For this review, take the finished solid that the model builds, in its own axes (mm). A direction names the side the tool comes from. Give positions to 0.01 mm unless a question says otherwise; leave off trailing zeros. Loops run counter-clockwise (first coordinate to the right, second up) from the corner with the lowest first, then second, coordinate; pieces in that order, holes last. Notation, with made-up numbers: (17.5, -33.5) - (33.5, -33.5) arc R34 cw to (33.5, 5.5) - close; hole circle Ø9 at (33, 37). An arc over 180 degrees is marked (long way). Use CSV: the item, a comma, the result in double quotes. Start each with the question number.
1. For pin 1 (0.9 mm diameter, centred on x = 34, z = 1.5, fed in from -Y); pin 2 (1.5 mm diameter, centred on y = 3, z = 2, fed in from +X); pin 3 (0.9 mm diameter, centred on y = -29.5, z = 2, fed in from -X); pin 4 (8 mm diameter, centred on x = 16, y = 2.5, fed in from -Z), all flat-tipped, find the tip position at first contact; note any pin that passes through.
2. Take a section at C-C on y = 10.5. Give the boundary of the cut face in (x, z), plus the area to 3 significant figures.
3. For faces 4 (the flat face through (36, 7.5, 1)), 5 (the flat face through (-20, 30, 1)), 6 (the flat face through (-7.5, -52, 1)), 7 (the flat face through (25, -7, 1)), 8 (the flat face through (-35, -30, 1)), list the 3-axis set-ups (+Z, -Z, +X, -X, +Y, -Y) from which the entire face can be reached by the end or side of a thin tool; tool diameter is ignored.
4. Take a section at D-D on x = 20. Give the boundary of the cut face in (y, z).
5. Mouldability with a two-part tool opening along X and no side actions: class faces 1 (the flat face through (-37, -22.5, 1)), 2 (the flat face through (-5, -8, 1)), 3 (the flat face through (35, 0, 1)) as pulls with the +X half, pulls with the -X half, needs draft (parallel to the pull), parting line crosses it, or undercut.
6. Wall thickness on line 1 (X direction, y = 12, z = 1.1); line 2 (X direction, y = -30, z = 1.15); line 3 (X direction, y = 27, z = 0.65): over which ranges is each line inside the solid? List them lowest first.
7. Take a section at B-B on x = -20. Give the boundary of the cut face in (y, z).
8. Take a section at A-A on y = -5. Give the boundary of the cut face in (x, z), plus the area to 3 significant figures.
```python
from build123d import *

# Parameters (mm, degrees)
BOSS_EXTRUDE1_DEPTH = 3


with BuildPart() as part:
    # Sketch1 → Boss-Extrude1 (new body)
    with BuildSketch(Plane.XY):
        Polygon((35, 50), (-3, 30), (-38, 30), (-38, 7.5), (-35, 7.5), (-35, -7.5), (-38, -7.5), (-38, -22.5), (-35, -22.5), (-35, -37.5), (-38, -37.5), (-38, -50), (-27.5, -50), (-27.5, -53), (-7.5, -53), (-7.5, -50), (7.5, -50), (7.5, -53), (27.5, -53), (27.5, -50), (38, -50), (38, -37.5), (35, -37.5), (35, -22.5), (38, -22.5), (38, -7.5), (35, -7.5), (35, 7.5), (38, 7.5), (38, 22.5), (35, 22.5), (35, 37.5), (38, 37.5), (38, 50), align=None)
        with BuildLine():
            Line((-15, 20), (-15, -35))
            ThreePointArc((-15, -35), (-20, -40), (-25, -35))
            Line((-25, -35), (-25, 20))
            ThreePointArc((-25, 20), (-20, 25), (-15, 20))
        make_face(mode=Mode.SUBTRACT)
        with BuildLine():
            ThreePointArc((5, -35), (0, -40), (-5, -35))
            Line((-5, -35), (-5, 20))
            ThreePointArc((-5, 20), (0, 25), (5, 20))
            Line((5, 20), (5, -35))
        make_face(mode=Mode.SUBTRACT)
        with BuildLine():
            ThreePointArc((25, -35), (20, -40), (15, -35))
            Line((15, -35), (15, 20))
            ThreePointArc((15, 20), (20, 25), (25, 20))
            Line((25, 20), (25, -35))
        make_face(mode=Mode.SUBTRACT)
    extrude(amount=BOSS_EXTRUDE1_DEPTH)


solid = part.part
```
Check result:
1,pin 1,"stops at y = -50"
1,pin 2,"stops at x = 35"
1,pin 3,"stops at x = -35"
1,pin 4,"stops at z = 0"
2,outline,"(-38, 0) - (-25, 0) - (-25, 3) - (-38, 3) - close; (-15, 0) - (-5, 0) - (-5, 3) - (-15, 3) - close; (5, 0) - (15, 0) - (15, 3) - (5, 3) - close; (25, 0) - (38, 0) - (38, 3) - (25, 3) - close"
2,area,"138 mm²"
3,face 4,"+Z, -Z, +X"
3,face 5,"+Z, -Z, -X, +Y"
3,face 6,"+Z, -Z, -Y"
3,face 7,"+Z, -Z"
3,face 8,"+Z, -Z, -X"
4,outline,"(-53, 0) - (-40, 0) - (-40, 3) - (-53, 3) - close; (25, 0) - (42.11, 0) - (42.11, 3) - (25, 3) - close"
5,face 1,"needs draft"
5,face 2,"undercut"
5,face 3,"pulls with the +X half"
6,line 1,"x = -38 to -25, -15 to -5, 5 to 15, 25 to 38"
6,line 2,"x = -35 to -25, -15 to -5, 5 to 15, 25 to 35"
6,line 3,"x = -38 to 35"
7,outline,"(-53, 0) - (-40, 0) - (-40, 3) - (-53, 3) - close; (25, 0) - (30, 0) - (30, 3) - (25, 3) - close"
8,outline,"(-35, 0) - (-25, 0) - (-25, 3) - (-35, 3) - close; (-15, 0) - (-5, 0) - (-5, 3) - (-15, 3) - close; (5, 0) - (15, 0) - (15, 3) - (5, 3) - close; (25, 0) - (35, 0) - (35, 3) - (25, 3) - close"
8,area,"120 mm²"
